Input: part model. Units: mm. Frame: model coordinates. A direction names the side the tool comes from. Give positions to 0.01 mm unless a question says otherwise; leave off trailing zeros. Loops run counter-clockwise (first coordinate to the right, second up) from the corner with the lowest first, then second, coordinate; pieces in that order, holes last.
from build123d import *

# Parameters (mm, degrees)
EXTRUDE1_DEPTH = 25
SKETCH2_R      = 9.9
EXTRUDE2_DEPTH = 14.5
SKETCH3_R      = 3
EXTRUDE3_DEPTH = 2.5
SKETCH4_R      = 1
EXTRUDE4_DEPTH = 3
SKETCH5_R      = 1
EXTRUDE5_DEPTH = 4
SKETCH6_R      = 3
EXTRUDE6_DEPTH = 2
SKETCH7_R      = 1.5
EXTRUDE7_DEPTH = 7.5
SKETCH8_W      = 0.5
SKETCH8_H      = 2.236067978
EXTRUDE8_DEPTH = 6.5


with BuildPart() as part:
    # Sketch1 → Extrude1 (new body)
    with BuildSketch(Plane.XY):
        with BuildLine():
            Line((-7.65, 6.440302788), (-7.65, -6.440302788))
            ThreePointArc((-7.65, -6.440302788), (0, -10), (7.65, -6.440302788))
            Line((7.65, -6.440302788), (7.65, 6.440302788))
            ThreePointArc((7.65, 6.440302788), (0, 10), (-7.65, 6.440302788))
        make_face()
    extrude(amount=EXTRUDE1_DEPTH)

    # Sketch2 → Extrude2 (add)
    with BuildSketch(Plane.XY.offset(25)):
        with Locations(Location((0, 0, 0), (0, 0, 140.599431246))):
            Circle(SKETCH2_R)
    extrude(amount=EXTRUDE2_DEPTH)

    # Sketch3 → Extrude3 (add)
    with BuildSketch(Plane(origin=(0, 0, 0), x_dir=(-1, 0, 0), z_dir=(0, 0, -1))):
        with Locations(Location((0, 0, 0), (0, 0, 180))):
            Circle(SKETCH3_R)
    extrude(amount=EXTRUDE3_DEPTH)

    # Sketch4 → Extrude4 (add)
    with BuildSketch(Plane(origin=(0, 0, -2.5), x_dir=(-1, 0, 0), z_dir=(0, 0, -1))):
        Circle(SKETCH4_R)
    extrude(amount=EXTRUDE4_DEPTH)

    # Sketch5 → Extrude5 (add)
    with BuildSketch(Plane(origin=(0, 0, 0), x_dir=(-1, 0, 0), z_dir=(0, 0, -1))):
        with Locations(Location((-2.65, 7.016231182, 0), (0, 0, 180))):
            Circle(SKETCH5_R)
        with Locations(Location((2.65, -7.016231182, 0), (0, 0, 180))):
            Circle(SKETCH5_R)
    extrude(amount=EXTRUDE5_DEPTH)

    # Sketch6 → Extrude6 (add)
    with BuildSketch(Plane.XY.offset(39.5)):
        with Locations((0, 4)):
            Circle(SKETCH6_R)
    extrude(amount=EXTRUDE6_DEPTH)

    # Sketch7 → Extrude7 (add)
    with BuildSketch(Plane.XY.offset(41.5)):
        with Locations((0, 4)):
            Circle(SKETCH7_R)
    extrude(amount=EXTRUDE7_DEPTH)

    # Sketch8 → Extrude8 (cut)
    with BuildSketch(Plane.XY.offset(49)):
        with Locations((1.25, 4)):
            Rectangle(SKETCH8_W, SKETCH8_H)
    extrude(amount=-EXTRUDE8_DEPTH, mode=Mode.SUBTRACT)


solid = part.part
(1) Cut plane D-D (y = 4). Return the cut outline in (x, z), and give its area (3 significant figures).
Values follow:
outline: (-9.06, 25) - (-7.65, 25) - (-7.65, 0) - (7.65, 0) - (7.65, 25) - (9.06, 25) - (9.06, 39.5) - (3, 39.5) - (3, 41.5) - (1.5, 41.5) - (1.5, 42.5) - (1, 42.5) - (1, 49) - (-1.5, 49) - (-1.5, 41.5) - (-3, 41.5) - (-3, 39.5) - (-9.06, 39.5) - close
area: 676 mm2
(2) Mould query, pull axis Y, two halves, no side actions, for faces 1 (the cylindrical face through (2.43, 7.99, -1.97)), 2 (the flat face through (0, 4, 49)), 3 (the cylindrical face through (2.86, -0.9, -1.23)), 4 (the cylindrical face through (0, -1, -4)). Classes: +Y half, -Y half, draft (parallel to the pull), parting line (faces both ways), or undercut.
Values follow:
face 1: undercut
face 2: draft
face 3: undercut
face 4: parting line
(3) Cut plane C-C (z = 19.5). Return the cut outline in (x, y).
Values follow:
outline: (-7.65, -6.44) arc R10 ccw to (7.65, -6.44) - (7.65, 6.44) arc R10 ccw to (-7.65, 6.44) - close
(4) Cut plane A-A (x = 0). Return the cut outline in (y, z).
Values follow:
outline: (-10, 0) - (-3, 0) - (-3, -2.5) - (-1, -2.5) - (-1, -5.5) - (1, -5.5) - (1, -2.5) - (3, -2.5) - (3, 0) - (10, 0) - (10, 25) - (9.9, 25) - (9.9, 39.5) - (7, 39.5) - (7, 41.5) - (5.5, 41.5) - (5.5, 49) - (2.5, 49) - (2.5, 41.5) - (1, 41.5) - (1, 39.5) - (-9.9, 39.5) - (-9.9, 25) - (-10, 25) - close
(5) Pin query (flat end, axial travel): pin 1 Ø8 at (y, z) = (3, 1) entering from -X; pin 2 Ø1.9 at (x, y) = (1, -9) entering from +Z; pin 3 Ø2 at (x, y) = (3, 7) entering from -Z. Return the tip coordinate at first contact, or that it passes through.
Values follow:
pin 1: stops at x = -7.65
pin 2: stops at z = 39.5
pin 3: stops at z = -4
(6) Cut plane B-B (y = 0). Return the cut outline in (x, z), and give its area (3 significant figures).
Values follow:
outline: (-9.9, 25) - (-7.65, 25) - (-7.65, 0) - (-3, 0) - (-3, -2.5) - (-1, -2.5) - (-1, -5.5) - (1, -5.5) - (1, -2.5) - (3, -2.5) - (3, 0) - (7.65, 0) - (7.65, 25) - (9.9, 25) - (9.9, 39.5) - (-9.9, 39.5) - close
area: 691 mm2
(7) Reachability of faces 5 (the flat face through (-1, -1, -2.5)), 6 (the flat face through (-7.65, 0, 12)), 7 (the flat face through (1.3, 2.7, 41.5)) from +Z, -Z, +X, -X, +Y, -Y: full face, straight path, thin tool, end or side. Return the list, or none.
Values follow:
face 5: -Z
face 6: -Z, -X, +Y, -Y
face 7: +Z
(8) Ray query, probe 1 along Z at (x, y) = (7.25, 0.75); probe 2 along Z at (x, y) = (8, 4.75); probe 3 along X at (y, z) = (-6, 2). Return the intervals inside material, ascending.
Values follow:
probe 1: z = 0 to 39.5
probe 2: z = 25 to 39.5
probe 3: x = -7.65 to 7.65
